Job drawing, mm, ordinate dimensions from the low corner. One solid piece. Coordinates: 2 decimals unless noted, no trailing zeros. Write each loop counter-clockwise with the first axis right and the second up, starting at its lowest first coordinate (ties: lowest second). Pieces come first, ordered by that corner, then holes. Notation, with made-up numbers: (46, -38.5) - (83, -38.5) arc R29 cw to (83, 0.5) - close; hole circle Ø6 at (10, -28). An arc over 180 degrees is marked (long way). Use one line per item in the form item = value. Start each with the question number.
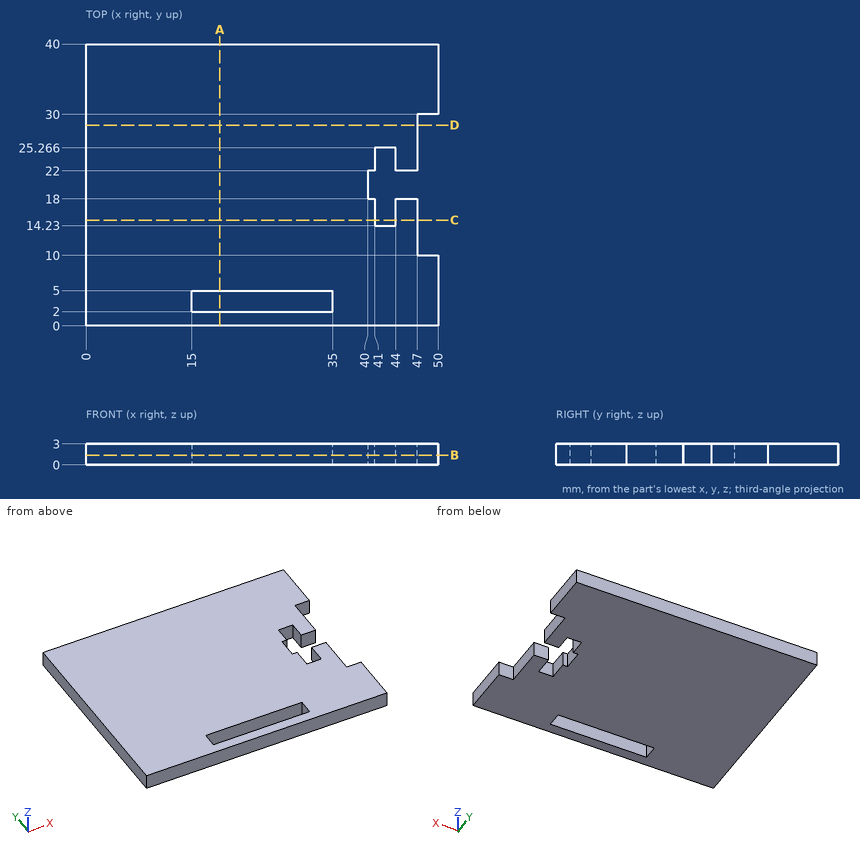
Q1. Slice it at C-C (y = 15). List the corners of the cut face in (x, z), plus the area to 3 significant figures.
Q2. Slice it at A-A (x = 19). List the corners of the cut face in (y, z).
Q3. Slice it at B-B (z = 1.4). List the corners of the cut face in (x, y).
Q4. Pin check, flat tips, straight feed: P1, Ø1.5, axis at y = 20, z = 1, coming from the +X side; P2, Ø6, axis at x = 24, y = 21, coming from the -Z side; P3, Ø1.5, axis at y = 28, z = 1, coming from the +X side. Stop position of each tip, or through.
Q5. Slice it at D-D (y = 28.5). List the corners of the cut face in (x, z).
Q6. Drill centre lines: probe 1 along Y at (x, z) = (16, 0.9); probe 2 along Y at (x, z) = (45.5, 2.7); probe 3 along X at (y, z) = (22.5, 2.5). Where is each one in solid material? Low to high.
Solution:
q1.outline = (0, 0) - (41, 0) - (41, 3) - (0, 3) - close; (44, 0) - (47, 0) - (47, 3) - (44, 3) - close
q1.area = 132 mm2
q2.outline = (0, 0) - (2, 0) - (2, 3) - (0, 3) - close; (5, 0) - (40, 0) - (40, 3) - (5, 3) - close
q3.outline = (0, 0) - (50, 0) - (50, 10) - (47, 10) - (47, 18) - (44, 18) - (44, 14.23) - (41, 14.23) - (41, 18) - (40, 18) - (40, 22) - (41, 22) - (41, 25.27) - (44, 25.27) - (44, 22) - (47, 22) - (47, 30) - (50, 30) - (50, 40) - (0, 40) - close; hole (15, 2) - (35, 2) - (35, 5) - (15, 5) - close
q4.P1 = 40
q4.P2 = 0
q4.P3 = 47
q5.outline = (0, 0) - (47, 0) - (47, 3) - (0, 3) - close
q6.probe_1 = 0 to 2, 5 to 40
q6.probe_2 = 0 to 18, 22 to 40
q6.probe_3 = 0 to 41, 44 to 47
